Job drawing, mm, ordinate dimensions from the low corner. One solid piece. Give positions to 0.01 mm unless a question says otherwise; leave off trailing zeros. Order: outer loops, then holes, each group sorted by start corner. A loop starts at its lowest first (then second) coordinate and runs counter-clockwise, first axis right, second up.
Item 1: Band-saw the part on C-C on x = 127.5. Give the cut face in (y, z), plus the area to 3 significant figures.
Item 2: Two-plate mould, pull along X, no slides. Class the marked faces 1, 2 and 3: released by +X, released by -X, zero draft, split by the parting line, or undercut.
Item 3: Flat gauge pin, fed straight in: P1, Ø1, axis at x = 112, z = 4.5, coming from the +Y side. Where does the tip first touch, or does it go through?
Item 4: Band-saw the part on B-B on z = 4.5. Give the cut face in (x, y).
Item 5: Band-saw the part on A-A on x = 35. Give the cut face in (y, z), plus the area to 3 significant figures.
Item 6: Band-saw the part on D-D on x = 83. Give the cut face in (y, z).
Item 7: Wall check: L1, parallel to X at y = 12.75, z = 6.5; L2, parallel to X at y = 23.5, z = 8.5; L3, parallel to X at y = 14, z = 8.75. Give the ranges that are in metal, low to high.
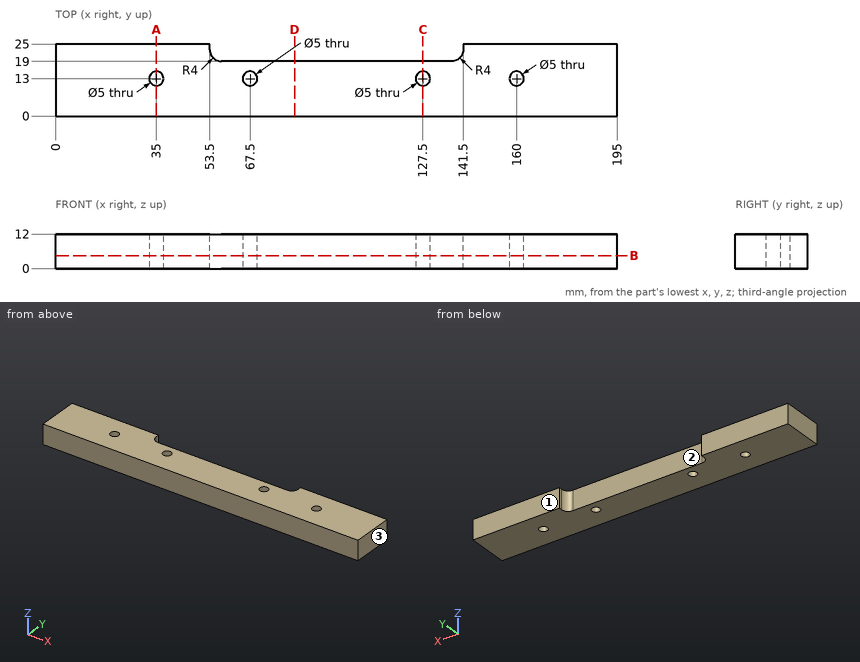
The answers:
1. outline: (0, 0) - (10.5, 0) - (10.5, 12) - (0, 12) - close; (15.5, 0) - (19, 0) - (19, 12) - (15.5, 12) - close
1. area: 168 mm2
2. face 1: zero draft
2. face 2: undercut
2. face 3: released by +X
3. P1: stops at y = 19
4. outline: (0, 0) - (195, 0) - (195, 25) - (141.5, 25) - (141.5, 23) arc R4 cw to (137.5, 19) - (57.5, 19) arc R4 cw to (53.5, 23) - (53.5, 25) - (0, 25) - close; hole circle Ø5 at (35, 13); hole circle Ø5 at (67.5, 13); hole circle Ø5 at (127.5, 13); hole circle Ø5 at (160, 13)
5. outline: (0, 0) - (10.5, 0) - (10.5, 12) - (0, 12) - close; (15.5, 0) - (25, 0) - (25, 12) - (15.5, 12) - close
5. area: 240 mm2
6. outline: (0, 0) - (19, 0) - (19, 12) - (0, 12) - close
7. L1: x = 0 to 32.51, 37.49 to 65.01, 69.99 to 125.01, 129.99 to 157.51, 162.49 to 195
7. L2: x = 0 to 53.5, 141.5 to 195
7. L3: x = 0 to 32.71, 37.29 to 65.21, 69.79 to 125.21, 129.79 to 157.71, 162.29 to 195
